```python
from build123d import *

# Parameters (mm, degrees)
SKETCH_1_R          = 16
EXTRUDE_1_DEPTH     = 5
SKETCH_2_R          = 6
CUT_EXTRUDE_1_DEPTH = 11
SKETCH_3_R          = 13.7
SKETCH_3_R_2        = 9.25
CUT_EXTRUDE_2_DEPTH = 0.5


with BuildPart() as part:
    # 草圖1 → 填料-伸長1 (new body, symmetric)
    with BuildSketch(Plane.XY):
        Circle(SKETCH_1_R)
    extrude(amount=EXTRUDE_1_DEPTH, both=True)

    # 草圖2 → 除料-伸長1 (cut, through all)
    with BuildSketch(Plane.XY.offset(5)):
        Circle(SKETCH_2_R)
    extrude(amount=-CUT_EXTRUDE_1_DEPTH, mode=Mode.SUBTRACT)

    # 草圖3 → 除料-伸長2 (cut)
    with BuildSketch(Plane.XY.offset(5)):
        Circle(SKETCH_3_R)
        Circle(SKETCH_3_R_2, mode=Mode.SUBTRACT)
    cut_extrude_2 = extrude(amount=-CUT_EXTRUDE_2_DEPTH, mode=Mode.SUBTRACT)

    # 鏡射1: 除料-伸長2 across plane
    add(cut_extrude_2.mirror(Plane.XY), mode=Mode.SUBTRACT)


solid = part.part
```
Design review of the part built by this model. Coordinates are the model's own, in mm. A direction names the side the tool comes from. Round coordinates to 2 decimals unless told otherwise and drop trailing zeros. Write each loop counter-clockwise with the first axis right and the second up, starting at its lowest first coordinate (ties: lowest second). Pieces come first, ordered by that corner, then holes.
Item 1: The part is to be moulded in two halves that separate along X. For faces 4 (the flat face through (12, 7, -5)), 5 (the cylindrical face through (-3.47, -15.62, 0.07)), 6 (the cylindrical face through (-2.01, -9.03, 4.75)), say which applies: +X half, -X half, draft (parallel to the pull), parting line (faces both ways), or undercut.
Item 2: Clearance check with flat-ended pins moving along their axes: pin 1 Ø6 at (x, z) = (4, 3.5) entering from +Y; pin 2 Ø1 at (y, z) = (-9, -4) entering from -X; pin 3 Ø2 at (x, z) = (10, 3) entering from -Y. State where each tip first meets the part, or that it passes through.
Item 3: We need section A-A on y = 0. Write out the cut boundary in (x, z), and give its area (3 significant figures).
Item 4: For faces 1 (the cylindrical face through (-10.097, 9.259, 4.754)), 2 (the flat face through (2, -6, -5)), 3 (the cylindrical face through (-10.097, 9.259, -4.754)), list the 3-axis set-ups (+Z, -Z, +X, -X, +Y, -Y) from which the entire face can be reached by the end or side of a thin tool; tool diameter is ignored.
Item 5: For probe 1 along Y at (x, z) = (0, 4.95); probe 2 along Y at (x, z) = (0, 2); probe 3 along Z at (x, y) = (-3, 13), list the stretches that pass through material, from the lowest coordinate up.
Item 6: We need section D-D on y = -10.5. Write out the cut boundary in (x, z).
Item 7: We need section C-C on z = -3.75. Write out the cut boundary in (x, y), and give its area (3 significant figures).
Returned:
1. face 4: draft
1. face 5: parting line
1. face 6: undercut
2. pin 1: stops at y = 15.97
2. pin 2: stops at x = -13.56
2. pin 3: stops at y = -13.23
3. outline: (-16, -5) - (-13.7, -5) - (-13.7, -4.5) - (-9.25, -4.5) - (-9.25, -5) - (-6, -5) - (-6, 5) - (-9.25, 5) - (-9.25, 4.5) - (-13.7, 4.5) - (-13.7, 5) - (-16, 5) - close; (6, -5) - (9.25, -5) - (9.25, -4.5) - (13.7, -4.5) - (13.7, -5) - (16, -5) - (16, 5) - (13.7, 5) - (13.7, 4.5) - (9.25, 4.5) - (9.25, 5) - (6, 5) - close
3. area: 191 mm2
4. face 1: +Z
4. face 2: -Z, +X, -X, +Y, -Y
4. face 3: -Z
5. probe 1: y = -16 to -13.7, -9.25 to -6, 6 to 9.25, 13.7 to 16
5. probe 2: y = -16 to -6, 6 to 16
5. probe 3: z = -4.5 to 4.5
6. outline: (-12.07, -5) - (-8.8, -5) - (-8.8, -4.5) - (8.8, -4.5) - (8.8, -5) - (12.07, -5) - (12.07, 5) - (8.8, 5) - (8.8, 4.5) - (-8.8, 4.5) - (-8.8, 5) - (-12.07, 5) - close
7. outline: circle Ø32 at (0, 0); hole circle Ø12 at (0, 0)
7. area: 691 mm2
